```python
from build123d import *

# Parameters (mm, degrees)
CUT_EXTRUDE_START        = 10
CUT_EXTRUDE_1_DEPTH      = 164.502052104
CUT_EXTRUDE_2_DEPTH      = 127.723636311
PATTERN_CIRCULAR_1_COUNT = 30
FILLET_2_R               = 1
CHAMFER_1_SIZE           = 1.5


with BuildPart() as part:
    # Эскиз1 → Повернуть1 (revolve)
    with BuildSketch(Plane.XY, mode=Mode.PRIVATE) as revolve_1_sk:
        Polygon((0, -12.5), (26, -12.5), (26, -15), (62, -15), (62, -18), (70, -18), (70, -28.8), (120, -28.8), (120, -15), (134, -15), (134, -12.5), (148, -12.5), (148, 0), (0, 0), align=None)
    revolve(revolve_1_sk.sketch.rotate(Axis((0, 0, 0), (1, 0, 0)), 270), axis=Axis((0, 0, 0), (1, 0, 0)))

    # Эскиз2 → Вырез-Повернуть1 (revolve, cut)
    with BuildSketch(Plane.XY, mode=Mode.PRIVATE) as cut_revolve_1_sk:
        Polygon((0, 4.25), (3.9, 2), (8.9, 2), (10.054700538, 0), (0, 0), align=None)
    cut_revolve_1 = revolve(cut_revolve_1_sk.sketch.rotate(Axis((0, 0, 0), (1, 0, 0)), 90), axis=Axis((0, 0, 0), (1, 0, 0)), mode=Mode.SUBTRACT)

    # Зеркальное отражение1: Вырез-Повернуть1 across plane
    add(cut_revolve_1.mirror(Plane.ZY.offset(-74)), mode=Mode.SUBTRACT)

    # Эскиз3 → Вырез-Вытянуть1 (cut, through all)
    with BuildSketch(Plane.XY.offset(CUT_EXTRUDE_START)):
        with BuildLine():
            Line((37, 4), (51, 4))
            ThreePointArc((51, 4), (55, 0), (51, -4))
            Line((51, -4), (37, -4))
            ThreePointArc((37, -4), (33, 0), (37, 4))
        make_face()
    extrude(amount=-CUT_EXTRUDE_1_DEPTH, mode=Mode.SUBTRACT)

    # Эскиз4 → Вырез-Вытянуть2 (cut, through all)
    with BuildSketch(Plane(origin=(120, 0, 0), x_dir=(0, 0, -1), z_dir=(1, 0, 0))):
        Polygon((5, 31.686751346), (-5, 31.686751346), (0, 23.026497308), align=None)
    cut_extrude_2 = extrude(amount=-CUT_EXTRUDE_2_DEPTH, mode=Mode.SUBTRACT)

    # Круговой массив1: Вырез-Вытянуть2 ×30 about axis
    pattern_circular_1_axis = Axis((0, 0, 0), (1, 0, 0))
    for i in range(1, PATTERN_CIRCULAR_1_COUNT):
        add(cut_extrude_2.rotate(pattern_circular_1_axis, i * 360 / PATTERN_CIRCULAR_1_COUNT), mode=Mode.SUBTRACT)

    # Скругление2
    fillet_2_edges = [part.edges().sort_by_distance(p)[0] for p in [
        (95, 22.523313095, -4.787477989),
        (95, 21.035752021, -9.365720217),
        (95, 26.92098276, -8.747157541),
        (95, 18.628827643, -13.53463553),
        (95, 24.514058382, -14.153198206),
        (95, 11.513248654, -19.941531629),
        (95, 16.638082356, -22.900355747),
        (95, 15.407734106, -17.112022323),
        (95, 21.035752021, -18.940676195),
        (95, 7.115578989, -21.899500312),
        (95, 11.513248654, -25.859179864),
        (95, 2.406924378, -22.900355747),
        (95, 5.885230739, -27.687833735),
        (95, -7.115578989, -21.899500312),
        (95, -5.885230739, -27.687833735),
        (95, -2.406924378, -22.900355747),
        (95, 0, -28.306396412),
        (95, -11.513248654, -19.941531629),
        (95, -11.513248654, -25.859179864),
        (95, -15.407734106, -17.112022323),
        (95, -16.638082356, -22.900355747),
        (95, -21.035752021, -9.365720217),
        (95, -24.514058382, -14.153198206),
        (95, -18.628827643, -13.53463553),
        (95, -21.035752021, -18.940676195),
        (95, -22.523313095, -4.787477989),
        (95, -26.92098276, -8.747157541),
        (95, -23.026497308, 0),
        (95, -28.15133101, -2.958824118),
        (95, -21.035752021, 9.365720217),
        (95, -26.92098276, 8.747157541),
        (95, -22.523313095, 4.787477989),
        (95, -28.15133101, 2.958824118),
        (95, -18.628827643, 13.53463553),
        (95, -24.514058382, 14.153198206),
        (95, -15.407734106, 17.112022323),
        (95, -21.035752021, 18.940676195),
        (95, -7.115578989, 21.899500312),
        (95, -11.513248654, 25.859179864),
        (95, -11.513248654, 19.941531629),
        (95, -16.638082356, 22.900355747),
        (95, -2.406924378, 22.900355747),
        (95, -5.885230739, 27.687833735),
        (95, 2.406924378, 22.900355747),
        (95, 0, 28.306396412),
        (95, 11.513248654, 19.941531629),
        (95, 11.513248654, 25.859179864),
        (95, 7.115578989, 21.899500312),
        (95, 5.885230739, 27.687833735),
        (95, 15.407734106, 17.112022323),
        (95, 16.638082356, 22.900355747),
        (95, 18.628827643, 13.53463553),
        (95, 21.035752021, 18.940676195),
        (95, 22.523313095, 4.787477989),
        (95, 26.92098276, 8.747157541),
        (95, 21.035752021, 9.365720217),
        (95, 24.514058382, 14.153198206),
        (95, 23.026497308, 0),
        (95, 28.15133101, 2.958824118),
        (95, 28.15133101, -2.958824118),
    ]]
    fillet(fillet_2_edges, radius=FILLET_2_R)

    # Фаска1
    chamfer_1_edges = [part.edges().sort_by_distance(p)[0] for p in [
        (148, 0, -12.5),
        (134, 0, -15),
        (62, 0, -18),
        (26, 0, -15),
        (0, 0, -12.5),
    ]]
    chamfer(chamfer_1_edges, length=CHAMFER_1_SIZE)


solid = part.part
```
Check sheet for the modelled part. Datum: model origin and axes. Units: mm. A direction names the side the tool comes from. Coordinates: 2 decimals unless noted, no trailing zeros. Loops run counter-clockwise (first coordinate to the right, second up) from the corner with the lowest first, then second, coordinate; pieces in that order, holes last.
1) Gauge pin test, flat ends, axial feed: pin 1 (3 mm diameter, centred on y = -10.5, z = 18.5, fed in from +X); pin 2 (1 mm diameter, centred on x = 105.5, z = 22, fed in from +Y); pin 3 (15.5 mm diameter, centred on x = 42.5, z = -6, fed in from +Y). Record the tip position at first contact, or that the pin passes through.
2) Sectioned sample at A-A (x = 31.5). Record the boundary of the cut face in (y, z).
3) Release check for a two-part mould opening along X. For faces 5 (the face through (66.796, -5.407, 17.169)), 6 (the face through (55, 0, -2)), 7 (the face through (134, 9, 9)) record: released by +X, released by -X, zero draft, split by the parting line, or undercut.
4) Material ranges on probe 1 along Y at (x, z) = (6, 0); probe 2 along X at (y, z) = (-21.5, -9); probe 3 along Z at (x, y) = (95, -23), recorded low to high.
5) Access from +Z, -Z, +X, -X, +Y, -Y to the whole of each face (thin tool, end or side, straight path). Record for faces 1 (the face through (0, 5, 0)), 2 (the face through (33, 0, -2)), 3 (the face through (6, 2, 0)), 4 (the face through (142, 2, 0)).
Check sheet entries:
1. pin 1: stops at x = 120
1. pin 2: stops at y = 16
1. pin 3: stops at y = 15
2. outline: circle Ø30 at (0, 0)
3. face 5: zero draft
3. face 6: undercut
3. face 7: released by +X
4. probe 1: y = -12.5 to -2, 2 to 12.5
4. probe 2: x = 70 to 120
4. probe 3: z = -13.71 to -12.07, -9.16 to 9.16, 12.07 to 13.71
5. face 1: +Z, -Z, -X, +Y, -Y
5. face 2: -Z
5. face 3: -X
5. face 4: +X
